Here's the drawing with two shaded views (mm, measured from the low corner). I have some questions. Coordinates: 2 decimals unless noted, no trailing zeros. Order: outer loops, then holes, each group sorted by start corner. A loop starts at its lowest first (then second) coordinate and runs counter-clockwise, first axis right, second up. Notation, with made-up numbers: (27, 16) -> (78, 16) arc R17 cw to (78, 45) -> close; hole circle Ø9 at (73.25, 41). An arc over 180 degrees is marked (long way). Answer in a Markdown table with one row per item. Add a question column.
1. We'd pull the mould along Z, two halves only. Please class the marked faces 1, 2, 3 and 4: pulls with the +Z half, pulls with the -Z half, needs draft (parallel to the pull), parting line crosses it, or undercut.
2. Imagine slicing it at D-D on y = 1. Write out the boundary of the cut face in (x, z).
3. Will this pin go through, and if not, where does the flat tip stop? pin 1 (4 mm diameter, centred on y = 2, z = 12, fed in from -X).
4. Imagine slicing it at C-C on x = 25. Write out the boundary of the cut face in (y, z), plus the area to 3 significant figures.
5. Imagine slicing it at B-B on y = 5. Write out the boundary of the cut face in (x, z).
6. If I drill on line 1 along X through (y, z) = (2.75, 7.25); line 2 along Y through (x, z) = (25, 9.75); line 3 along X through (y, z) = (3.5, 9.25), over which ranges is the centre line in solid material (lowest first)? Write a range as [from, to].
7. Imagine slicing it at A-A on z = 7.25. Write out the boundary of the cut face in (x, y).
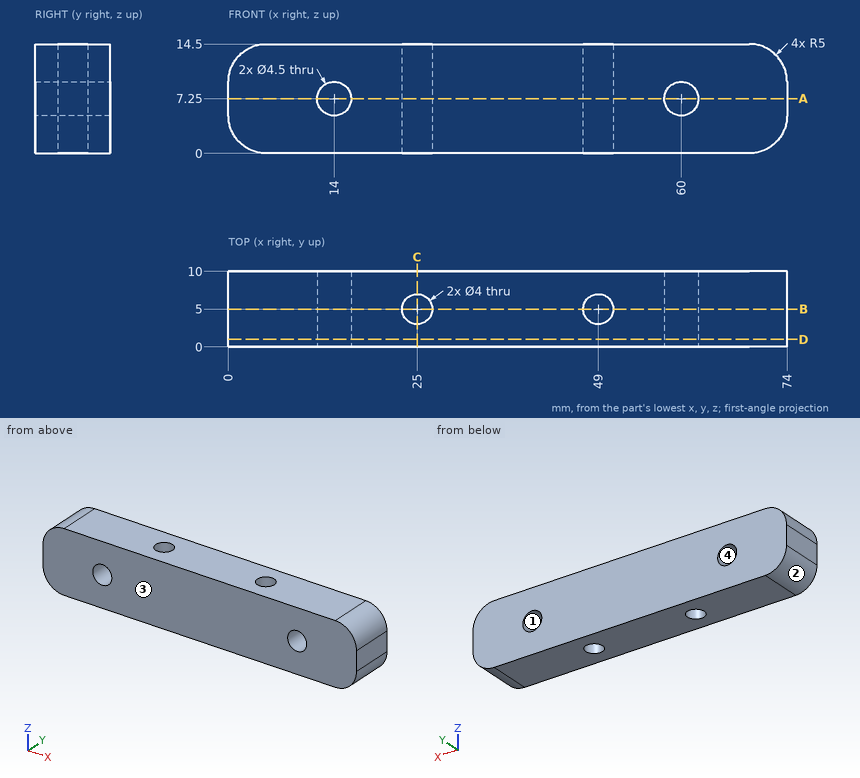
Answers follow:
| question | item | result |
|---|---|---|
| 1 | face 1 | undercut |
| 1 | face 2 | pulls with the -Z half |
| 1 | face 3 | needs draft |
| 1 | face 4 | undercut |
| 2 | outline | (0, 5) arc R5 ccw to (5, 0) -> (69, 0) arc R5 ccw to (74, 5) -> (74, 9.5) arc R5 ccw to (69, 14.5) -> (5, 14.5) arc R5 ccw to (0, 9.5) -> close; hole circle Ø4.5 at (14, 7.25); hole circle Ø4.5 at (60, 7.25) |
| 3 | pin 1 | stops at x = 0.03 |
| 4 | outline | (0, 0) -> (3, 0) -> (3, 14.5) -> (0, 14.5) -> close; (7, 0) -> (10, 0) -> (10, 14.5) -> (7, 14.5) -> close |
| 4 | area | 87.0 mm² |
| 5 | outline | (0, 5) arc R5 ccw to (5, 0) -> (23, 0) -> (23, 14.5) -> (5, 14.5) arc R5 ccw to (0, 9.5) -> close; (27, 0) -> (47, 0) -> (47, 14.5) -> (27, 14.5) -> close; (51, 0) -> (69, 0) arc R5 ccw to (74, 5) -> (74, 9.5) arc R5 ccw to (69, 14.5) -> (51, 14.5) -> close; hole circle Ø4.5 at (14, 7.25); hole circle Ø4.5 at (60, 7.25) |
| 6 | line 1 | x = [0, 11.75], [16.25, 57.75], [62.25, 74] |
| 6 | line 2 | y = [0, 3], [7, 10] |
| 6 | line 3 | x = [0, 12.97], [15.03, 23.68], [26.32, 47.68], [50.32, 58.97], [61.03, 74] |
| 7 | outline | (0, 0) -> (11.75, 0) -> (11.75, 10) -> (0, 10) -> close; (16.25, 0) -> (57.75, 0) -> (57.75, 10) -> (16.25, 10) -> close; (62.25, 0) -> (74, 0) -> (74, 10) -> (62.25, 10) -> close; hole circle Ø4 at (25, 5); hole circle Ø4 at (49, 5) |
